```python
from build123d import *

# Parameters (mm, degrees)
SKETCH_1_W          = 190
SKETCH_1_H          = 144
SKETCH_1_R          = 6
EXTRUDE_1_DEPTH     = 12
SKETCH_2_W          = 190
SKETCH_2_H          = 12
SKETCH_2_W_2        = 260
EXTRUDE_2_DEPTH     = 145
SKETCH_3_R          = 6
CUT_EXTRUDE_1_DEPTH = 239.589605809
SKETCH_4_R          = 6
EXTRUDE_3_DEPTH     = 6
SKETCH_5_W          = 10
SKETCH_5_H          = 100
EXTRUDE_4_DEPTH     = 145
SKETCH_6_W          = 25
SKETCH_6_H          = 20
EXTRUDE_5_DEPTH     = 145


with BuildPart() as part:
    # 草图1 → 凸台-拉伸1 (new body)
    with BuildSketch(Plane(origin=(0, 0, 0), x_dir=(1, 0, 0), z_dir=(0, 1, 0))):
        Rectangle(SKETCH_1_W, SKETCH_1_H)
        with Locations(Location((-57, 41, 0), (0, 0, 270))):
            Circle(SKETCH_1_R, mode=Mode.SUBTRACT)
        with Locations(Location((57, 41, 0), (0, 0, 270))):
            Circle(SKETCH_1_R, mode=Mode.SUBTRACT)
        with Locations(Location((-57, -2, 0), (0, 0, 270))):
            Circle(SKETCH_1_R, mode=Mode.SUBTRACT)
        with Locations(Location((57, -2, 0), (0, 0, 270))):
            Circle(SKETCH_1_R, mode=Mode.SUBTRACT)
    extrude(amount=EXTRUDE_1_DEPTH)

    # 草图2 → 凸台-拉伸2 (add)
    with BuildSketch(Plane(origin=(0, 12, 0), x_dir=(1, 0, 0), z_dir=(0, 1, 0))):
        with Locations((0, 66)):
            Rectangle(SKETCH_2_W, SKETCH_2_H)
        with Locations((0, -46)):
            Rectangle(SKETCH_2_W_2, SKETCH_2_H)
    extrude(amount=EXTRUDE_2_DEPTH)

    # 草图3 → 切除-拉伸1 (cut, through all)
    with BuildSketch(Plane.XY.offset(52)):
        with Locations((-30, 132)):
            Circle(SKETCH_3_R)
        with Locations((30, 132)):
            Circle(SKETCH_3_R)
        with BuildLine():
            Line((-17.5, 157), (17.5, 157))
            Line((17.5, 157), (17.5, 102))
            ThreePointArc((17.5, 102), (0, 84.5), (-17.5, 102))
            Line((-17.5, 102), (-17.5, 157))
        make_face()
    extrude(amount=-CUT_EXTRUDE_1_DEPTH, mode=Mode.SUBTRACT)

    # 草图4 → 凸台-拉伸3 (add)
    with BuildSketch(Plane(origin=(0, 0, 40), x_dir=(-1, 0, 0), z_dir=(0, 0, -1))):
        with BuildLine():
            Line((-17.5, 142), (-39.5, 142))
            Line((-39.5, 142), (-39.5, 102))
            ThreePointArc((-39.5, 102), (0, 62.5), (39.5, 102))
            Line((39.5, 102), (39.5, 142))
            Line((39.5, 142), (17.5, 142))
            Line((17.5, 142), (17.5, 102))
            ThreePointArc((17.5, 102), (0, 84.5), (-17.5, 102))
            Line((-17.5, 102), (-17.5, 142))
        make_face()
        with Locations(Location((-30, 132, 0), (0, 0, 180))):
            Circle(SKETCH_4_R, mode=Mode.SUBTRACT)
        with Locations(Location((30, 132, 0), (0, 0, 180))):
            Circle(SKETCH_4_R, mode=Mode.SUBTRACT)
    extrude(amount=EXTRUDE_3_DEPTH)

    # 草图5 → 凸台-拉伸4 (add)
    with BuildSketch(Plane(origin=(0, 157, 0), x_dir=(1, 0, 0), z_dir=(0, 1, 0))):
        with Locations((-90, 10)):
            Rectangle(SKETCH_5_W, SKETCH_5_H)
        with Locations((90, 10)):
            Rectangle(SKETCH_5_W, SKETCH_5_H)
    extrude(amount=-EXTRUDE_4_DEPTH)

    # 草图6 → 凸台-拉伸5 (add)
    with BuildSketch(Plane(origin=(0, 12, 0), x_dir=(1, 0, 0), z_dir=(0, 1, 0))):
        with Locations((-82.5, -62)):
            Rectangle(SKETCH_6_W, SKETCH_6_H)
        with Locations((82.5, -62)):
            Rectangle(SKETCH_6_W, SKETCH_6_H)
    extrude(amount=EXTRUDE_5_DEPTH)


solid = part.part
```
The model under review builds one solid part; all positions refer to its coordinate system, in mm. A direction names the side the tool comes from. Round coordinates to 2 decimals unless told otherwise and drop trailing zeros. Loops run counter-clockwise (first coordinate to the right, second up) from the corner with the lowest first, then second, coordinate; pieces in that order, holes last. Notation, with made-up numbers: (39, 44.25) - (92, 44.25) arc R28 ccw to (92, 78.25) - close; hole circle Ø8 at (89.25, 22). An arc over 180 degrees is marked (long way). Write each question's results on one line, items separated by ' | '. Start each with the question number.
Q1. Take a section at A-A on x = -57. Give the boundary of the cut face in (y, z).
Q2. Take a section at B-B on z = -41. Give the boundary of the cut face in (x, y), plus the area to 3 significant figures.
Q3. Tool access review of faces 1 (the flat face through (-1, 12, 62)), 2 (the flat face through (39.5, 122, 37)), 3 (the flat face through (17.5, 129, 43)): name each direction out of +Z, -Z, +X, -X, +Y, -Y from which nothing blocks a thin tool from reaching the whole face with its end or side.
Q4. Draft analysis for pull direction Z (two halves, no side actions). For faces 4 (the flat face through (-20, 67, 40)), 5 (the flat face through (-1, 77, -72)), 6 (the flat face through (-113, 12, 46)), state which applies: pulls with the +Z half, pulls with the -Z half, needs draft (parallel to the pull), parting line crosses it, or undercut.
Q5. Take a section at D-D on z = -63. Give the boundary of the cut face in (x, y).
Q6. Insertion check: P1, Ø10, axis at y = 115.5, z = 66.5, coming from the -X side; P2, Ø10, axis at x = -11, z = 55, coming from the +Y side; P3, Ø13, axis at x = -115.5, z = 46.5, coming from the -Y side; P4, Ø11, axis at x = -57, z = -41, coming from the +Y side (3 decimals). Each pin has a flat end and moves straight along its axis. Give the tip position at first contact, or say it passes through.
Q7. Wall thickness on line 1 along X through (y, z) = (132, 38); line 2 along Z through (x, y) = (7, 58.5); line 3 along X through (y, z) = (85.5, -30.5): over which ranges is each line inside the solid? List them lowest first. Write a range as [from, to].
Data:
1) outline: (0, -72) - (157, -72) - (157, -60) - (12, -60) - (12, -47) - (0, -47) - close; (0, -35) - (12, -35) - (12, -4) - (0, -4) - close; (0, 8) - (12, 8) - (12, 40) - (157, 40) - (157, 52) - (12, 52) - (12, 72) - (0, 72) - close
2) outline: (-95, 0) - (-63, 0) - (-63, 12) - (-85, 12) - (-85, 157) - (-95, 157) - close; (-51, 0) - (51, 0) - (51, 12) - (-51, 12) - close; (63, 0) - (95, 0) - (95, 157) - (85, 157) - (85, 12) - (63, 12) - close | area: 4,890 mm²
3) face 1: +Z, +Y | face 2: +Y | face 3: +Z, -Z, +Y
4) face 4: undercut | face 5: pulls with the -Z half | face 6: needs draft
5) outline: (-95, 0) - (95, 0) - (95, 157) - (17.5, 157) - (17.5, 102) arc R17.5 cw to (-17.5, 102) - (-17.5, 157) - (-95, 157) - close; hole circle Ø12 at (-30, 132); hole circle Ø12 at (30, 132)
6) P1: stops at x = -95 | P2: stops at y = 92.99 | P3: stops at y = 12 | P4: passes through
7) line 1: x = [-95, -85], [-39.5, -36], [-24, -17.5], [17.5, 24], [36, 39.5], [85, 95] | line 2: z = [-72, -60], [40, 52] | line 3: x = [-95, -85], [85, 95]
